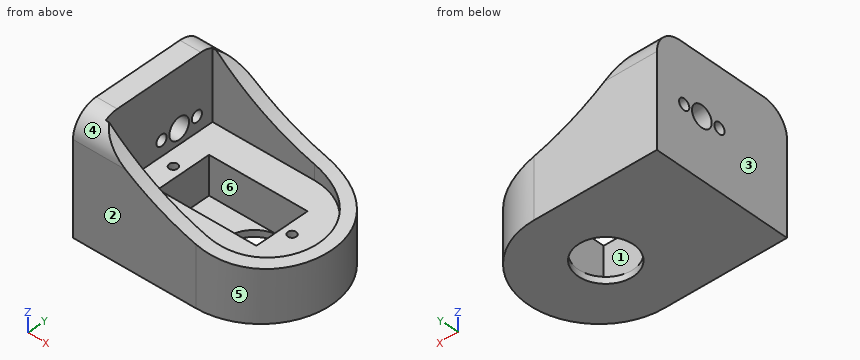
Autodesk Inventor part; units mm, degrees
ref_plane "YZ Plane" through (0, 0, 0) normal (1, 0, 0) x (0, 1, 0)
ref_plane "XZ Plane" through (0, 0, 0) normal (0, 1, 0) x (-1, 0, 0)
ref_plane "XY Plane" through (0, 0, 0) normal (0, 0, 1) x (1, 0, 0)
sketch "Sketch1" plane through (0, 0, 0) normal (0, 0, 1) x (1, 0, 0)
  line L0 (0, 0) -> (115, 0)
  line L1 (115, 0) -> (115, 84)
  line L2 (115, 84) -> (0, 84)
  line L3 (0, 84) -> (0, 0)
  line L4 (115, 42) -> (0, 42) construction
  circle A0 centre (69, 42) radius 16.5
  arc A1 (73, 0) -> (73, 84) centre (73, 42) ccw
  dimension "d0" = 115
  dimension "d1" = 84
  dimension "d2" = 33
  dimension "d3" = 46
extrude "Extrusion1" add sketch "Sketch1" along normal blind 70 contours L3 L2 A1 L0
sketch "Sketch2" plane through (0, 0, 70) normal (0, 0, 1) x (1, 0, 0)
  arc A0 (73, 0) -> (73, 84) centre (73, 42) ccw
  line L0 (73, 84) -> (0, 84)
  line L1 (0, 84) -> (0, 0)
  line L2 (0, 0) -> (73, 0)
  arc A1 (73, 0) -> (73, 84) centre (73, 42) ccw
  line L3 (12.5, 76.5) -> (73, 76.5)
  arc A2 (73, 7.5) -> (73, 76.5) centre (73, 42) ccw
  line L4 (73, 7.5) -> (12.5, 7.5)
  line L5 (12.5, 76.5) -> (12.5, 7.5)
  dimension "d6" = 7.5
  dimension "d7" = 12.5
extrude "Extrusion2" cut sketch "Sketch2" against normal blind 43.3 contours L3 A2 L4 L5
sketch "Sketch3" plane through (0, 0, 0) normal (0, 1, 0) x (-1, 0, 0)
  line L0 (0, 0) -> (0, 70) construction
  line L1 (0, 30.5) -> (-115.317, 30.5) construction
  line L2 (-73, 0) -> (-115, 0) construction
  line L3 (-73, 0) -> (0, 0) construction
  line L4 (-12.5, 0) -> (-12.5, 70) construction
  line L5 (-107.817, 30.5) -> (-107.817, 0) construction
  arc A0 (-115.317, 30.5) -> (-12.5, 70) centre (-111.567, 174.3032) ccw
  line L6 (-12.5, 70) -> (-115.317, 70)
  line L7 (-115.317, 30.5) -> (-115.317, 70)
  dimension "d10" = 30.5
  dimension "d11" = 12.5
  dimension "d12" = 7.5
extrude "Extrusion3" cut sketch "Sketch3" along normal through all
fillet "Fillet1" radius 15 2 edges at (6.25, 0, 70) (6.25, 84, 70)
sketch "Sketch4" plane through (12.5, 7.5, 26.7) normal (1, 0, 0) x (0, 0, -1)
  line L0 (-9.0174, -7.5) -> (-28.3, -7.5) construction
  line L1 (-9, -7.5) -> (-9, 76.5) construction
  line L2 (26.7, 76.5) -> (-28.3, 76.5) construction
  line L3 (0, 0) -> (0, 69) construction
  circle A0 centre (-9, 47.5) radius 6.35
  circle A1 centre (-9, 58.9) radius 3.3
  circle A2 centre (-9, 36.1) radius 3.3
  point P0 (26.7, -7.5)
  dimension "d16" = 9
  dimension "d17" = 12.7
  dimension "d18" = 29
  dimension "d19" = 6.6
  dimension "d20" = 11.4
  dimension "d21" = 6.6
  dimension "d22" = 11.4
extrude "Extrusion4" cut sketch "Sketch4" against normal through all
sketch "Sketch5" plane through (0, 0, 26.7) normal (0, 0, 1) x (1, 0, 0)
  circle A0 centre (69, 42) radius 16.5 construction
  line L0 (85.5, 42) -> (85.5, 58.5) construction
  line L1 (69, 58.5) -> (85.5, 58.5) construction
  line L2 (85.5, 58.5) -> (27, 58.5)
  line L3 (27, 58.5) -> (27, 25.5)
  line L4 (27, 25.5) -> (85.5, 25.5)
  line L5 (85.5, 25.5) -> (85.5, 58.5)
  point P0 (0, 0)
  dimension "d25" = 58.5
extrude "Extrusion5" cut sketch "Sketch5" against normal blind 22.8
sketch "Sketch6" plane through (0, 0, 26.7) normal (0, 0, 1) x (1, 0, 0)
  line L0 (27, 25.5) -> (27, 58.5) construction
  line L1 (27, 42) -> (12.5, 42) construction
  line L2 (12.5, 46.9) -> (12.5, 40.3) construction
  circle A0 centre (21, 42) radius 2.5
  line L3 (85.5, 25.5) -> (27, 25.5) construction
  line L4 (56.25, 25.5) -> (56.25, 58.5) construction
  circle A1 centre (91.5, 42) radius 2.5
  point P0 (0, 0)
  dimension "d28" = 5
  dimension "d29" = 6
extrude "Extrusion6" cut sketch "Sketch6" against normal blind 20.3
properties part number "Final Arm 03"
Build history of the part. All positions in model axes, mm. Face numbers are marked on the shaded views. A direction names the side the tool comes from. Round coordinates to 2 decimals unless told otherwise and drop trailing zeros. Write each loop counter-clockwise with the first axis right and the second up, starting at its lowest first coordinate (ties: lowest second). Pieces come first, ordered by that corner, then holes. Notation, with made-up numbers: (-21.75, 0) -> (26.25, 0) arc R24 cw to (26.25, 36) -> close; hole circle Ø9 at (4.25, 16.5). An arc over 180 degrees is marked (long way). Use one line per item in the form item = value.
Q1. Drop flat-ended pins along their axis: P1, Ø4, axis at y = 66.4, z = 35.7, coming from the +X side; P2, Ø18, axis at x = 76, y = 51.5, coming from the +Z side; P3, Ø13, axis at y = 54, z = 51.5, coming from the +X side; P4, Ø7, axis at y = 47, z = 13, coming from the +X side. Give the stop position or say it passes through.
Conclusion:
P1 = through
P2 = 26.7
P3 = 12.5
P4 = 114.97
Q2. Band-saw the part on C-C, the plane y = 66.4. Write the cut outline in (x, z).
Conclusion:
outline = (0, 0) -> (107.19, 0) -> (107.19, 30.52) arc R143.85 cw to (97.39, 31.15) -> (97.39, 26.7) -> (12.5, 26.7) -> (12.5, 32.4) -> (0, 32.4) -> close; (0, 39) -> (12.5, 39) -> (12.5, 70) -> (0, 70) -> close
Q3. Two-plate mould, pull along Y, no slides. Class the marked faces 3, 4, 5 and 6: released by +Y, released by -Y, zero draft, split by the parting line, or undercut.
Conclusion:
face_3 = zero draft
face_4 = released by -Y
face_5 = split by the parting line
face_6 = undercut
Q4. Band-saw the part on B-B, the plane z = 10. Write the cut outline in (x, y).
Conclusion:
outline = (0, 0) -> (73, 0) arc R42 ccw to (73, 84) -> (0, 84) -> close; hole circle Ø5 at (21, 42); hole (27, 25.5) -> (85.5, 25.5) -> (85.5, 58.5) -> (27, 58.5) -> close; hole circle Ø5 at (91.5, 42)
Q5. Drill centre lines: L1, parallel to Y at x = 8, z = 35.7; L2, parallel to Y at x = 5, z = 35; L3, parallel to Y at x = 21, z = 50. Where is each one in solid material? Low to high.
Conclusion:
L1 = 0 to 40.3, 46.9 to 48.65, 61.35 to 63.1, 69.7 to 84
L2 = 0 to 40.38, 46.82 to 48.69, 61.31 to 63.18, 69.62 to 84
L3 = 0 to 7.5, 76.5 to 84
Q6. Tool access for the marked faces 1 and 2: list every direction of +Z, -Z, +X, -X, +Y, -Y with a clear straight run to the whole face (end or side of a thin tool).
Conclusion:
face_1 = +Z
face_2 = +Z, -Z, +X, -X, -Y
Q7. Band-saw the part on A-A, the plane x = 79. Write the cut outline in (y, z), then the cut area to 3 significant figures.
Conclusion:
outline = (0.43, 0) -> (28.88, 0) -> (28.88, 3.9) -> (25.5, 3.9) -> (25.5, 26.7) -> (8.03, 26.7) -> (8.03, 34.19) -> (0.43, 34.19) -> close; (55.12, 0) -> (83.57, 0) -> (83.57, 34.19) -> (75.97, 34.19) -> (75.97, 26.7) -> (58.5, 26.7) -> (58.5, 3.9) -> (55.12, 3.9) -> close
area = 1,480 mm²
Q8. Band-saw the part on D-D, the plane z = 37.5. Write the cut outline in (x, y), then the cut area to 3 significant figures.
Conclusion:
outline = (0, 0) -> (67.09, 0) -> (67.09, 7.5) -> (12.5, 7.5) -> (12.5, 40.83) -> (0, 40.83) -> close; (0, 46.37) -> (12.5, 46.37) -> (12.5, 48.91) -> (0, 48.91) -> close; (0, 61.09) -> (12.5, 61.09) -> (12.5, 63.63) -> (0, 63.63) -> close; (0, 69.17) -> (12.5, 69.17) -> (12.5, 76.5) -> (67.09, 76.5) -> (67.09, 84) -> (0, 84) -> close
area = 1,580 mm²
